Here's the drawing with two shaded views (mm, measured from the low corner). I have some questions. Round coordinates to 2 decimals unless told otherwise and drop trailing zeros. Write each loop counter-clockwise with the first axis right and the second up, starting at its lowest first coordinate (ties: lowest second). Pieces come first, ordered by that corner, then holes. Notation, with made-up numbers: M 66.25,59 L 77.25,59 A12 cw 77.25,71 Z; hole C -33.5,-4 d7. An arc over 180 degrees is marked long. Write item = value, one per line. Start each with the question number.
(1) I want a section at D-D (y = 3). List the corners of the cut face in (x, z) for me.
(2) I want a section at C-C (x = 7). List the corners of the cut face in (y, z) for me, and give its area (3 significant figures).
(3) I want a section at A-A (y = 43). List the corners of the cut face in (x, z) for me, and give its area (3 significant figures).
(4) I need wall thicknesses on line 1 along X through (y, z) = (26.5, 1.55); line 2 along Y through (x, z) = (6.2, 1.5); line 3 along Y through (x, z) = (4.5, 0.35). Which ranges of each line are inside material? Lowest first, please.
(5) Will these pins go through, and if not, where does the flat tip stop? pin 1 Ø1 at (x, y) = (15, 41.5) entering from -Z; pin 2 Ø1 at (y, z) = (5.5, 1) entering from +X.
(6) I want a section at B-B (z = 0.75). List the corners of the cut face in (x, y) for me, and give its area (3 significant figures).
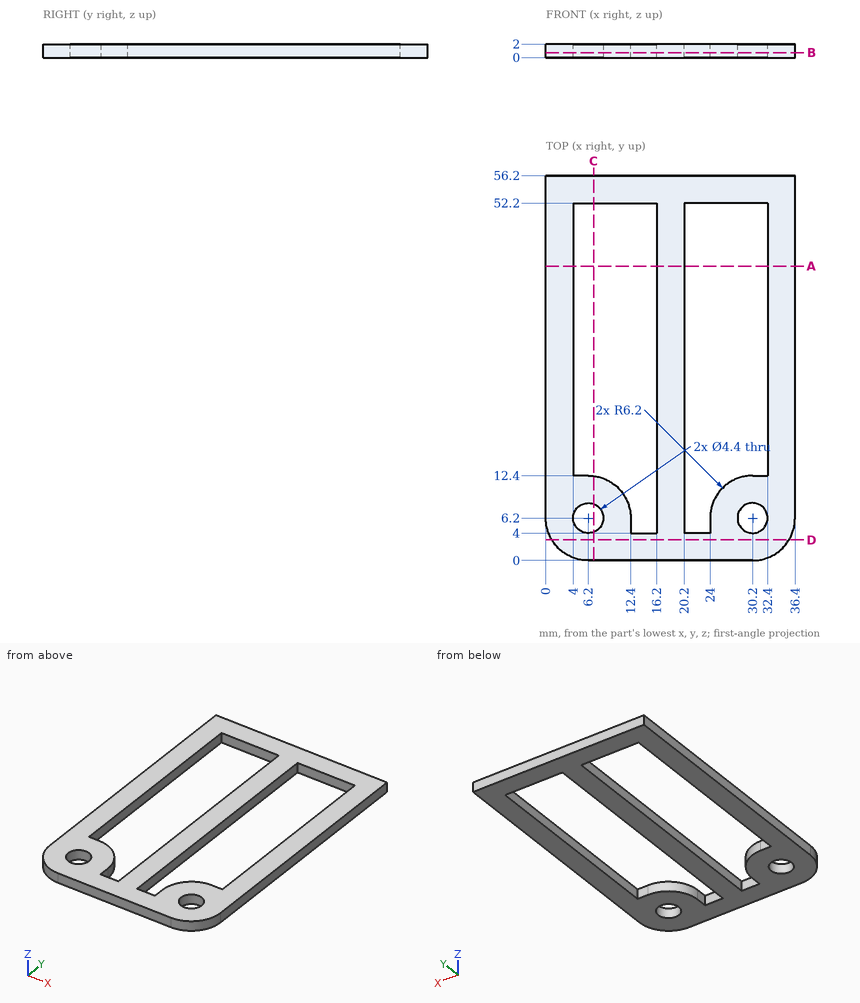
Returned:
q1.outline = M 0.89,0 L 35.51,0 L 35.51,2 L 0.89,2 Z
q2.outline = M 0,0 L 4.15,0 L 4.15,2 L 0,2 Z; M 8.25,0 L 12.35,0 L 12.35,2 L 8.25,2 Z; M 52.2,0 L 56.2,0 L 56.2,2 L 52.2,2 Z
q2.area = 24.5 mm²
q3.outline = M 0,0 L 4,0 L 4,2 L 0,2 Z; M 16.2,0 L 20.2,0 L 20.2,2 L 16.2,2 Z; M 32.4,0 L 36.4,0 L 36.4,2 L 32.4,2 Z
q3.area = 24.0 mm²
q4.line_1 = 0 to 4, 16.2 to 20.2, 32.4 to 36.4
q4.line_2 = 0 to 4, 8.4 to 12.4, 52.2 to 56.2
q4.line_3 = 0.24 to 4.8, 7.6 to 12.4, 52.2 to 56.2
q5.pin_1 = through
q5.pin_2 = 36.4
q6.outline = M 0,6.2 A6.2 ccw 6.2,0 L 30.2,0 A6.2 ccw 36.4,6.2 L 36.4,56.2 L 0,56.2 Z; hole C 6.2,6.2 d4.4; hole M 4,12.4 L 6.2,12.4 A6.2 cw 12.4,6.2 L 12.4,4 L 16.2,4 L 16.2,52.2 L 4,52.2 Z; hole M 20.2,4 L 24,4 L 24,6.2 A6.2 cw 30.2,12.4 L 32.4,12.4 L 32.4,52.2 L 20.2,52.2 Z; hole C 30.2,6.2 d4.4
q6.area = 947 mm²
